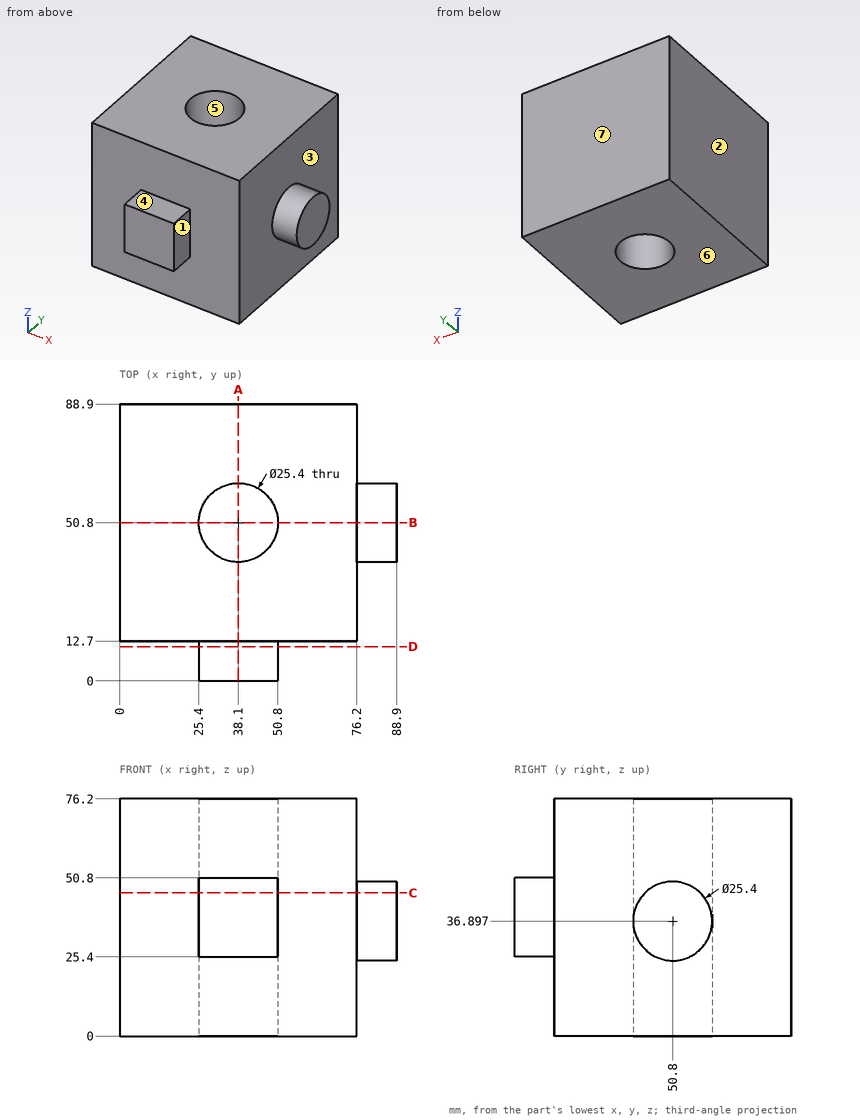
The figure shows three views and two pictorial views of one solid part (mm, origin at its lowest corner). Answer the questions. A direction names the side the tool comes from. Coordinates: 2 decimals unless noted, no trailing zeros. Write each loop counter-clockwise with the first axis right and the second up, starting at its lowest first coordinate (ties: lowest second). Pieces come first, ordered by that corner, then holes.
1. Flat-ended cylindrical pins translate along their axes: pin 1 (6.5 mm diameter, centred on x = 32.5, y = 7.5, fed in from +Z); pin 2 (6.5 mm diameter, centred on y = 5, z = 41, fed in from +X); pin 3 (12 mm diameter, centred on x = 10, z = 29.5, fed in from -Y); pin 4 (20.5 mm diameter, centred on x = 38.1, y = 50.8, fed in from +Z). Find the tip coordinate at first contact, or state that the pin passes through.
Results list:
pin 1: stops at z = 50.8
pin 2: stops at x = 50.8
pin 3: stops at y = 12.7
pin 4: passes through
2. The part is cut by section C-C, the plane z = 46. Write down the section's boundary in (x, y).
Results list:
outline: (0, 12.7) - (25.4, 12.7) - (25.4, 0) - (50.8, 0) - (50.8, 12.7) - (76.2, 12.7) - (76.2, 41.94) - (88.9, 41.94) - (88.9, 59.66) - (76.2, 59.66) - (76.2, 88.9) - (0, 88.9) - close; hole circle Ø25.4 at (38.1, 50.8)
3. The part is cut by section B-B, the plane y = 50.8. Write down the section's boundary in (x, z), and give its area (3 significant figures).
Results list:
outline: (0, 0) - (25.4, 0) - (25.4, 76.2) - (0, 76.2) - close; (50.8, 0) - (76.2, 0) - (76.2, 24.2) - (88.9, 24.2) - (88.9, 49.6) - (76.2, 49.6) - (76.2, 76.2) - (50.8, 76.2) - close
area: 4,190 mm2
4. For the marked faces 1, 2, 3 and 4, determine the directions among +Z, -Z, +X, -X, +Y, -Y from which every point of the face is accessible in a straight line to the end or side of a thin tool.
Results list:
face 1: +Z, -Z, +X, -Y
face 2: +Z, -Z, -X, +Y, -Y
face 3: +X
face 4: +Z, +X, -X, -Y
5. For a pull along Y with two mould halves and no side action, classify the marked faces 5, 6 and 7 as +Y half, -Y half, draft (parallel to the pull), parting line (faces both ways), or undercut.
Results list:
face 5: undercut
face 6: draft
face 7: +Y half
6. The part is cut by section D-D, the plane y = 11. Write down the section's boundary in (x, z).
Results list:
outline: (25.4, 25.4) - (50.8, 25.4) - (50.8, 50.8) - (25.4, 50.8) - close
7. Consider line 1 along Y through (x, z) = (38, 37); line 2 along Y through (x, z) = (38, 16); line 3 along X through (y, z) = (50, 22). Determine where each line is inside the solid, lowest interval first.
Results list:
line 1: y = 0 to 38.1, 63.5 to 88.9
line 2: y = 12.7 to 38.1, 63.5 to 88.9
line 3: x = 0 to 25.43, 50.77 to 76.2
8. The part is cut by section A-A, the plane x = 38.1. Write down the section's boundary in (y, z).
Results list:
outline: (0, 25.4) - (12.7, 25.4) - (12.7, 0) - (38.1, 0) - (38.1, 76.2) - (12.7, 76.2) - (12.7, 50.8) - (0, 50.8) - close; (63.5, 0) - (88.9, 0) - (88.9, 76.2) - (63.5, 76.2) - close
